Geometry: final body of the model. Coordinates: model frame, mm. Face numbers are marked on the shaded views. A direction names the side the tool comes from. Round coordinates to 2 decimals unless told otherwise and drop trailing zeros. Loops run counter-clockwise (first coordinate to the right, second up) from the corner with the lowest first, then second, coordinate; pieces in that order, holes last. Notation, with made-up numbers: (16, -30) - (49, -30) arc R33 ccw to (49, -2) - close; hole circle Ø1 at (74.25, -20.5). An arc over 180 degrees is marked (long way). Answer as a JSON object with one key per item and string values. Group by question number.
Item 1: Draft query along Z for the marked faces 4 and 5. Return one class per face: released by +Z, released by -Z, zero draft, split by the parting line, or undercut.
Item 2: Reachability of the marked faces 1, 2 and 3 from +Z, -Z, +X, -X, +Y, -Y: full face, straight path, thin tool, end or side. Return the list, or none.
Item 3: First-contact query: pin 1 (0.9 mm diameter, centred on x = -9, z = 99.5, fed in from -Y); pin 2 (2.5 mm diameter, centred on y = 8, z = 202.5, fed in from -X); pin 3 (2.5 mm diameter, centred on x = -15, y = 5, fed in from +Z). Flat tips, straight axial feed; report the tip coordinate or a pass-through.
Item 4: Section C-C (y = 10.75). Return the cut outline in (x, z).
Item 5: Section A-A (z = 22.5). Return the cut outline in (x, y).
Item 6: Section B-B (x = 4.5). Return the cut outline in (y, z).
Item 7: Section D-D (y = -0.5). Count the separate pieces of the cut face and the enclosed holes in it, plus the area to 3 significant figures.
Item 8: Line query: line 1 (X direction, y = 3.25, z = 44.5); line 2 (X direction, y = -5, z = 169.5). Output: solid intervals per line, ascending.
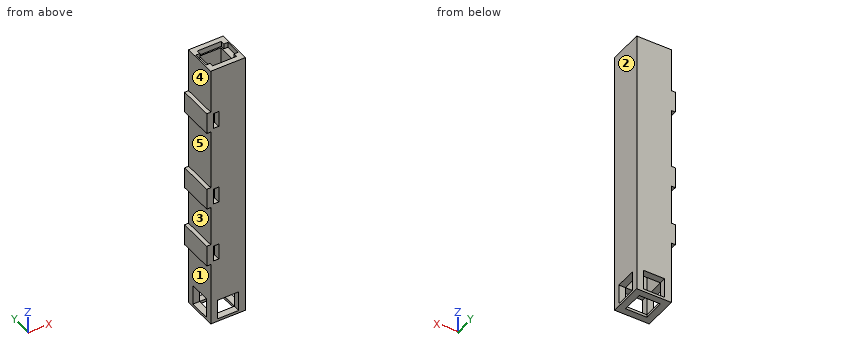
```python
from build123d import *

# Parameters (mm, degrees)
F0_W      = 26
F0_H      = 26
F0_W_2    = 16
F0_H_2    = 16
F1_DEPTH  = 2
F2_DEPTH  = 200
F3_W      = 26
F3_H      = 26
F3_W_2    = 18
F3_H_2    = 18
F4_DEPTH  = 4
F6_DEPTH  = 25
F7_W      = 3
F7_H      = 16
F8_DEPTH  = 26
F9_W      = 4
F9_H      = 12
F10_DEPTH = 20
F11_W     = 16
F11_H     = 15
F12_DEPTH = 40
F13_W     = 16
F13_H     = 15
F14_DEPTH = 40
F15_W     = 4
F15_H     = 12
F16_DEPTH = 20
F17_W     = 3
F17_H     = 12
F18_DEPTH = 4


with BuildPart() as f1:
    # F0 (on Top) → F1 (new body)
    with BuildSketch(Plane.XY):
        Rectangle(F0_W, F0_H)
        Rectangle(F0_W_2, F0_H_2, mode=Mode.SUBTRACT)
        Rectangle(F0_W_2, F0_H_2)
    extrude(amount=F1_DEPTH)

    # F0 (on Top) → F2 (join)
    with BuildSketch(Plane.XY):
        Rectangle(F0_W, F0_H)
        Rectangle(F0_W_2, F0_H_2, mode=Mode.SUBTRACT)
    extrude(amount=F2_DEPTH)

    # F3 (on face) → F4 (join)
    with BuildSketch(Plane.XY.offset(200)):
        Rectangle(F3_W, F3_H)
        Rectangle(F3_W_2, F3_H_2, mode=Mode.SUBTRACT)
    extrude(amount=F4_DEPTH)

    # F0 (on Top) → F6 (cut)
    with BuildSketch(Plane.XY):
        Rectangle(F0_W_2, F0_H_2)
    extrude(amount=F6_DEPTH, mode=Mode.SUBTRACT)

    # F7 (on face) → F8 (join)
    with BuildSketch(Plane.XZ.offset(13)):
        with Locations((-14.5, 163)):
            Rectangle(F7_W, F7_H)
        with Locations((-14.5, 102)):
            Rectangle(F7_W, F7_H)
        with Locations((-14.5, 56)):
            Rectangle(F7_W, F7_H)
    extrude(amount=-F8_DEPTH)

    # F9 (on face) → F10 (cut)
    with BuildSketch(Plane.XZ.offset(13)):
        with Locations((-9, 163)):
            Rectangle(F9_W, F9_H)
    extrude(amount=-F10_DEPTH, mode=Mode.SUBTRACT)

    # F11 (on face) → F12 (cut)
    with BuildSketch(Plane.XZ.offset(13)):
        with Locations((0, 9.5)):
            Rectangle(F11_W, F11_H)
    extrude(amount=-F12_DEPTH, mode=Mode.SUBTRACT)

    # F13 (on face) → F14 (cut)
    with BuildSketch(Plane.YZ.offset(13)):
        with Locations((0, 9.5)):
            Rectangle(F13_W, F13_H)
    extrude(amount=-F14_DEPTH, mode=Mode.SUBTRACT)

    # F15 (on face) → F16 (cut)
    with BuildSketch(Plane.XZ.offset(13)):
        with Locations((-9, 102)):
            Rectangle(F15_W, F15_H)
        with Locations((-9, 56)):
            Rectangle(F15_W, F15_H)
    extrude(amount=-F16_DEPTH, mode=Mode.SUBTRACT)

    # F17 (on face) → F18 (cut)
    with BuildSketch(Plane.XY.offset(204)):
        with Locations((-10.5, 0)):
            Rectangle(F17_W, F17_H)
        with Locations((10.5, 0)):
            Rectangle(F17_W, F17_H)
    extrude(amount=-F18_DEPTH, mode=Mode.SUBTRACT)


solid = f1.part
```
Values:
{
 "1": {"face 4": "zero draft", "face 5": "undercut"},
 "2": {"face 1": "-Z, -X, +Y, -Y", "face 2": "+Z, -Z, +X, +Y, -Y", "face 3": "-X, +Y, -Y"},
 "3": {"pin 1": "stops at y = 7", "pin 2": "stops at x = -13", "pin 3": "stops at z = 171"},
 "4": {"outline": "(-16, 48) - (-13, 48) - (-13, 0) - (13, 0) - (13, 204) - (-13, 204) - (-13, 171) - (-16, 171) - (-16, 155) - (-13, 155) - (-13, 110) - (-16, 110) - (-16, 94) - (-13, 94) - (-13, 64) - (-16, 64) - close; hole (-8, 2) - (8, 2) - (8, 17) - (-8, 17) - close"},
 "5": {"outline": "(-13, -13) - (13, -13) - (13, 13) - (-13, 13) - close; hole (-8, -8) - (8, -8) - (8, 8) - (-8, 8) - close"},
 "6": {"outline": "(-13, 0) - (-8, 0) - (-8, 2) - (-13, 2) - close; (-13, 17) - (-8, 17) - (-8, 200) - (-9, 200) - (-9, 204) - (-13, 204) - close; (8, 0) - (13, 0) - (13, 2) - (8, 2) - close; (8, 17) - (13, 17) - (13, 204) - (9, 204) - (9, 200) - (8, 200) - close"},
 "7": {"separate pieces": "4", "enclosed holes": "0", "area": "1,890 mm^2"},
 "8": {"line 1": "x = -13 to -8, 8 to 13", "line 2": "x = -16 to -8, 8 to 13"}
}
